For this review, take the finished solid that the model builds, in its own axes (mm). Face numbers are marked on the shaded views. Coordinates: 2 decimals unless noted, no trailing zeros. Loops run counter-clockwise (first coordinate to the right, second up) from the corner with the lowest first, then second, coordinate; pieces in that order, holes last. Notation, with made-up numbers: M 1.5,-33 L 25.5,-33 A22 cw 25.5,-15 Z; hole C -1.75,-38.75 d5. An arc over 180 degrees is marked long. Use one line per item in the form item = value.
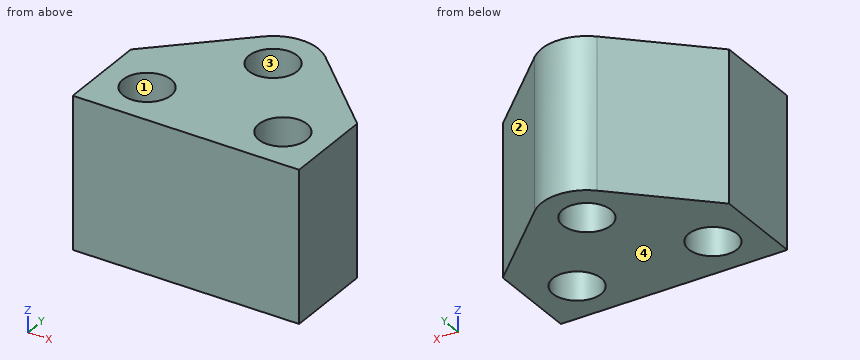
```python
from build123d import *

# Parameters (mm, degrees)
SKETCH1_R           = 1.6
BOSS_EXTRUDE1_DEPTH = 10


with BuildPart() as part:
    # Sketch1 → Boss-Extrude1 (new body)
    with BuildSketch(Plane.XY):
        with BuildLine():
            Line((-7.5, 6), (-2.068965517, 11.172413793))
            ThreePointArc((-2.068965517, 11.172413793), (0, 12), (2.068965517, 11.172413793))
            Line((2.068965517, 11.172413793), (7.5, 6))
            Line((7.5, 6), (7.5, 0))
            Line((7.5, 0), (-7.5, 0))
            Line((-7.5, 0), (-7.5, 6))
        make_face()
        with Locations((0, 9)):
            Circle(SKETCH1_R, mode=Mode.SUBTRACT)
        with Locations((-4.5, 3)):
            Circle(SKETCH1_R, mode=Mode.SUBTRACT)
        with Locations(Location((4.5, 3, 0), (0, 0, 180))):
            Circle(SKETCH1_R, mode=Mode.SUBTRACT)
    extrude(amount=BOSS_EXTRUDE1_DEPTH)


solid = part.part
```
1. Consider section B-B on y = 3. Write out the cut boundary in (x, z).
Computed values:
outline = M -7.5,0 L -6.1,0 L -6.1,10 L -7.5,10 Z; M -2.9,0 L 2.9,0 L 2.9,10 L -2.9,10 Z; M 6.1,0 L 7.5,0 L 7.5,10 L 6.1,10 Z
2. Draft analysis for pull direction Y (two halves, no side actions). For the marked faces 1, 2, 3 and 4, state which applies: +Y half, -Y half, draft (parallel to the pull), parting line (faces both ways), or undercut.
Computed values:
face_1 = undercut
face_2 = +Y half
face_3 = undercut
face_4 = draft
3. Consider section A-A on x = 0. Write out the cut boundary in (y, z), plus the area to 3 significant figures.
Computed values:
outline = M 0,0 L 7.4,0 L 7.4,10 L 0,10 Z; M 10.6,0 L 12,0 L 12,10 L 10.6,10 Z
area = 88.0 mm2
4. Wall thickness on line 1 along Y through (x, z) = (0, 2.5); line 2 along X through (y, z) = (2.25, 3); line 3 along X through (y, z) = (4, 8.5): over which ranges is each line inside the solid? List them lowest first. Write a range as from..to.
Computed values:
line_1 = 0..7.4, 10.6..12
line_2 = -7.5..-5.91, -3.09..3.09, 5.91..7.5
line_3 = -7.5..-5.75, -3.25..3.25, 5.75..7.5
5. For pin 1 Ø1.9 at (x, y) = (4.5, 3) entering from -Z, flat-tipped, find the tip position at first contact; note if it passes through.
Computed values:
pin_1 = through
6. Consider section D-D on y = 9. Write out the cut boundary in (x, z), plus the area to 3 significant figures.
Computed values:
outline = M -4.35,0 L -1.6,0 L -1.6,10 L -4.35,10 Z; M 1.6,0 L 4.35,0 L 4.35,10 L 1.6,10 Z
area = 55.0 mm2
7. Consider section C-C on z = 9. Write out the cut boundary in (x, y).
Computed values:
outline = M -7.5,0 L 7.5,0 L 7.5,6 L 2.07,11.17 A3 ccw -2.07,11.17 L -7.5,6 Z; hole C -4.5,3 d3.2; hole C 0,9 d3.2; hole C 4.5,3 d3.2
